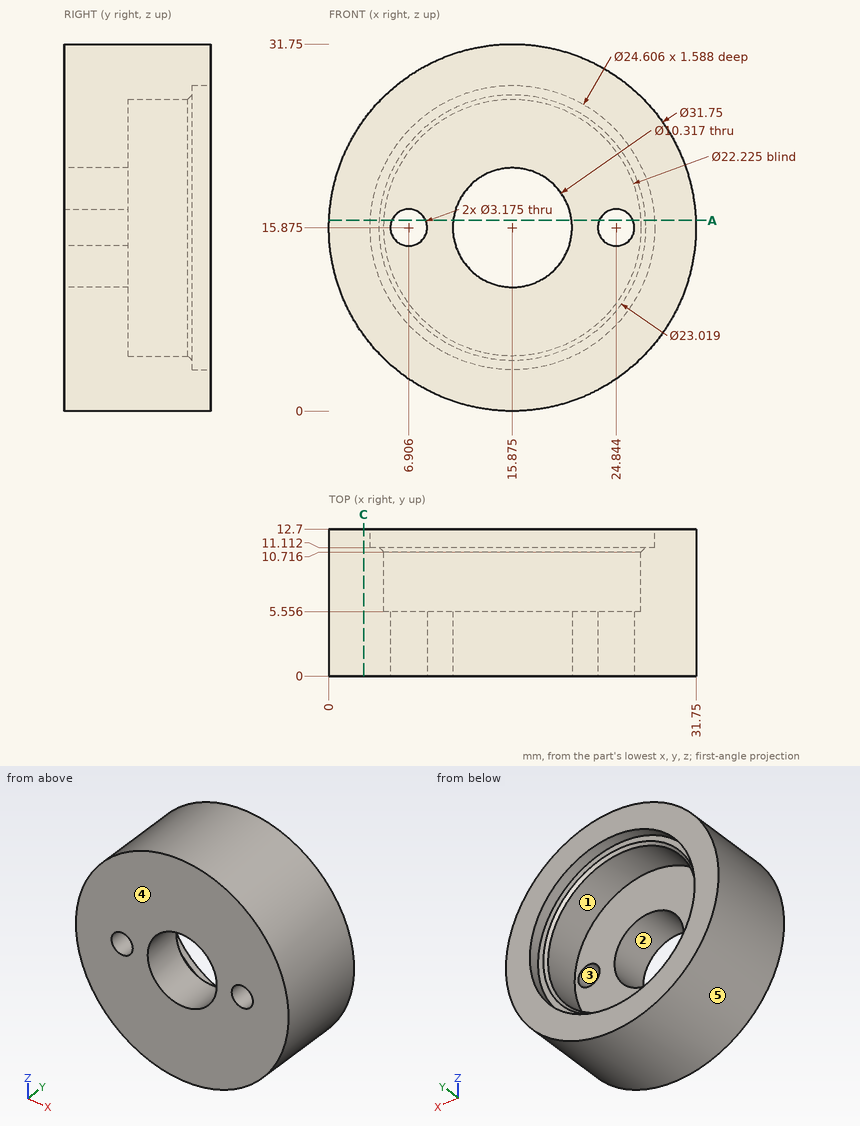
Could you check a few things on this drawing? It's one solid part, dimensions in mm from its lowest x, y, z. A direction names the side the tool comes from. Coordinates: 2 decimals unless noted, no trailing zeros. Order: outer loops, then holes, each group sorted by start corner. A loop starts at its lowest first (then second) coordinate and runs counter-clockwise, first axis right, second up. Notation, with made-up numbers: M -5,46 L 15,46 A33 ccw 15,85 Z; hole C 86,-4 d7. An arc over 180 degrees is marked long. Answer as CSV lines item,"result".
(1) I'm going to push flat-ended pins straight in: pin 1 (3.5 mm diameter, centred on x = 6.91, z = 15.88, fed in from +Y); pin 2 (4 mm diameter, centred on y = 7, z = 24.5, fed in from +X); pin 3 (6 mm diameter, centred on y = 1.5, z = 27, fed in from -X). Where does each tip first touch, or does it pass through?
Geometry check:
pin 1,"y = 5.56"
pin 2,"x = 30.3"
pin 3,"x = 2.24"
(2) If we mould it in two halves opening along Z, with no side actions, what happens to the marked faces 3, 4 and 5? For each: released by +Z, released by -Z, zero draft, split by the parting line, or undercut.
Geometry check:
face 3,"undercut"
face 4,"zero draft"
face 5,"split by the parting line"
(3) Please list where these lines run through material, in increasing order: L1, parallel to X at y = 1.75, z = 16.5 (1 decimal); L2, parallel to X at y = 7.75, z = 10 (1 decimal); L3, parallel to X at y = 6.25, z = 16.
Geometry check:
L1,"0 to 5.4, 8.4 to 10.8, 21 to 23.4, 26.3 to 31.7"
L2,"1.1 to 6.4, 25.3 to 30.6"
L3,"0 to 4.76, 26.99 to 31.75"
(4) Suppose I cut it at C-C on x = 3. Please give me the cut outline in (y, z).
Geometry check:
outline,"M 0,6.59 L 12.7,6.59 L 12.7,25.16 L 0,25.16 Z"
(5) On a 3-axis mill with a long thin cutter (end or side, diameter ignored), from which of +Z, -Z, +X, -X, +Y, -Y can I reach the whole of each face in a straight line? I mean the marked faces 1 and 2. Say none if no direction works.
Geometry check:
face 1,"+Y"
face 2,"+Y, -Y"
(6) Suppose I cut it at A-A on z = 16.5. Count the separate pieces of the cut face and the enclosed holes in it, plus the area to 3 significant figures.
Geometry check:
separate pieces,"4"
enclosed holes,"0"
area,"151 mm^2"
